Geometry: final body of the model. Coordinates: model frame, mm. Coordinates: 2 decimals unless noted, no trailing zeros. Write each loop counter-clockwise with the first axis right and the second up, starting at its lowest first coordinate (ties: lowest second). Pieces come first, ordered by that corner, then holes.
from build123d import *

# Parameters (mm, degrees)
SKETCH1_W           = 50
SKETCH1_H           = 20
SKETCH1_R           = 1.75
BOSS_EXTRUDE1_DEPTH = 1.6
SKETCH3_R           = 0.375
CUT_EXTRUDE1_DEPTH  = 2.6


with BuildPart() as part:
    # Sketch1 → Boss-Extrude1 (new body)
    with BuildSketch(Plane(origin=(0, 0, 0), x_dir=(1, 0, 0), z_dir=(0, 1, 0))):
        with Locations((25, 10)):
            Rectangle(SKETCH1_W, SKETCH1_H)
        with Locations((3, 17)):
            Circle(SKETCH1_R, mode=Mode.SUBTRACT)
        with Locations((47, 3)):
            Circle(SKETCH1_R, mode=Mode.SUBTRACT)
        with Locations((3, 3)):
            Circle(SKETCH1_R, mode=Mode.SUBTRACT)
        with Locations((47, 17)):
            Circle(SKETCH1_R, mode=Mode.SUBTRACT)
    extrude(amount=BOSS_EXTRUDE1_DEPTH)

    # Sketch3 → Cut-Extrude1 (cut, through all)
    with BuildSketch(Plane(origin=(0, 1.6, 0), x_dir=(1, 0, 0), z_dir=(0, 1, 0))):
        with Locations((8.25, 0.75)):
            Circle(SKETCH3_R)
        with Locations((9.75, 0.75)):
            Circle(SKETCH3_R)
        with Locations((9.75, 5.5)):
            Circle(SKETCH3_R)
        with Locations((9.75, 14.5)):
            Circle(SKETCH3_R)
        with Locations((13.25, 0.75)):
            Circle(SKETCH3_R)
        with Locations((14.75, 0.75)):
            Circle(SKETCH3_R)
        with Locations((14.75, 14.5)):
            Circle(SKETCH3_R)
        with Locations((14.75, 5.5)):
            Circle(SKETCH3_R)
        with Locations((18.25, 0.75)):
            Circle(SKETCH3_R)
        with Locations((19.75, 0.75)):
            Circle(SKETCH3_R)
        with Locations((19.75, 14.5)):
            Circle(SKETCH3_R)
        with Locations((19.75, 5.5)):
            Circle(SKETCH3_R)
        with Locations((23.25, 0.75)):
            Circle(SKETCH3_R)
        with Locations((24.75, 0.75)):
            Circle(SKETCH3_R)
        with Locations((24.75, 14.5)):
            Circle(SKETCH3_R)
        with Locations((24.75, 5.5)):
            Circle(SKETCH3_R)
        with Locations((28.25, 0.75)):
            Circle(SKETCH3_R)
        with Locations((29.75, 0.75)):
            Circle(SKETCH3_R)
        with Locations((29.75, 14.5)):
            Circle(SKETCH3_R)
        with Locations((29.75, 5.5)):
            Circle(SKETCH3_R)
        with Locations((33.25, 0.75)):
            Circle(SKETCH3_R)
        with Locations((34.75, 0.75)):
            Circle(SKETCH3_R)
        with Locations((34.75, 14.5)):
            Circle(SKETCH3_R)
        with Locations((34.75, 5.5)):
            Circle(SKETCH3_R)
        with Locations((38.25, 0.75)):
            Circle(SKETCH3_R)
        with Locations((39.75, 0.75)):
            Circle(SKETCH3_R)
        with Locations((39.75, 14.5)):
            Circle(SKETCH3_R)
        with Locations((39.75, 5.5)):
            Circle(SKETCH3_R)
    extrude(amount=-CUT_EXTRUDE1_DEPTH, mode=Mode.SUBTRACT)


solid = part.part
Item 1: Section C-C, the plane y = 0.9. State how many separate pieces and enclosed holes the cut face has, plus the area to 3 significant figures.
Derived:
separate pieces: 1
enclosed holes: 32
area: 949 mm2
Item 2: Pin query (flat end, axial travel): pin 1 (2 mm diameter, centred on x = 21, z = -10.5, fed in from -Y). Return the tip coordinate at first contact, or that it passes through.
Derived:
pin 1: stops at y = 0
Item 3: Section A-A, the plane x = 3. Output: boundary loops of the cut face in (y, z), plus the area to 3 significant figures.
Derived:
outline: (0, -20) - (1.6, -20) - (1.6, -18.75) - (0, -18.75) - close; (0, -15.25) - (1.6, -15.25) - (1.6, -4.75) - (0, -4.75) - close; (0, -1.25) - (1.6, -1.25) - (1.6, 0) - (0, 0) - close
area: 20.8 mm2
Item 4: Material intervals for probe 1 along Z at (x, y) = (39.75, 0.95) (3 decimals); probe 2 along X at (y, z) = (0.8, -15.75); probe 3 along Z at (x, y) = (28.25, 0.6) (3 decimals), sorted ascending.
Derived:
probe 1: z = -20 to -14.875, -14.125 to -5.875, -5.125 to -1.125, -0.375 to 0
probe 2: x = 0 to 1.78, 4.22 to 45.78, 48.22 to 50
probe 3: z = -20 to -1.125, -0.375 to 0
Item 5: Pull-direction query (Z, two-part tool) for faces 1 (the flat face through (25, 1, 0)), 2 (the cylindrical face through (3.81, 0.79, -1.45)), 3 (the flat face through (25, 1.6, -10)); classes: released by +Z, released by -Z, zero draft, split by the parting line, or undercut.
Derived:
face 1: released by +Z
face 2: undercut
face 3: zero draft
Item 6: Section B-B, the plane z = -17. Output: boundary loops of the cut face in (x, y).
Derived:
outline: (0, 0) - (1.25, 0) - (1.25, 1.6) - (0, 1.6) - close; (4.75, 0) - (45.25, 0) - (45.25, 1.6) - (4.75, 1.6) - close; (48.75, 0) - (50, 0) - (50, 1.6) - (48.75, 1.6) - close
